from build123d import *

# Parameters (mm, degrees)
ESTRUSIONE_ESTRUSIONE1_DEPTH = 1
ESTRUSIONE_ESTRUSIONE2_DEPTH = 1.5
SCHIZZO4_W                   = 20.34
SCHIZZO4_H                   = 2.54
TAGLIO_ESTRUSIONE1_DEPTH     = 1.5
SCHIZZO5_R                   = 1.25
TAGLIO_ESTRUSIONE2_DEPTH     = 10


with BuildPart() as part:
    # Schizzo2 → Estrusione-Estrusione1 (new body)
    with BuildSketch(Plane(origin=(0, 0, 0), x_dir=(1, 0, 0), z_dir=(0, 1, 0))):
        with BuildLine():
            Line((-3, 0), (-31, 0))
            ThreePointArc((-31, 0), (-33.121320344, 0.878679656), (-34, 3))
            Line((-34, 3), (-34, 47))
            ThreePointArc((-34, 47), (-33.121320344, 49.121320344), (-31, 50))
            Line((-31, 50), (-3, 50))
            ThreePointArc((-3, 50), (-0.878679656, 49.121320344), (0, 47))
            Line((0, 47), (0, 3))
            ThreePointArc((0, 3), (-0.878679656, 0.878679656), (-3, 0))
        make_face()
        with BuildLine():
            Line((-27, 43.75), (-7, 43.75))
            ThreePointArc((-7, 43.75), (-3.464466094, 42.285533906), (-2, 38.75))
            Line((-2, 38.75), (-2, 11.45))
            ThreePointArc((-2, 11.45), (-3.464466094, 7.914466094), (-7, 6.45))
            Line((-7, 6.45), (-27, 6.45))
            ThreePointArc((-27, 6.45), (-30.535533906, 7.914466094), (-32, 11.45))
            Line((-32, 11.45), (-32, 38.75))
            ThreePointArc((-32, 38.75), (-30.535533906, 42.285533906), (-27, 43.75))
        make_face(mode=Mode.SUBTRACT)
    extrude(amount=ESTRUSIONE_ESTRUSIONE1_DEPTH)

    # Schizzo3 → Estrusione-Estrusione2 (add)
    with BuildSketch(Plane(origin=(0, 1, 0), x_dir=(1, 0, 0), z_dir=(0, 1, 0))):
        with BuildLine():
            Line((-30, 52), (-4, 52))
            ThreePointArc((-4, 52), (0.242640687, 50.242640687), (2, 46))
            Line((2, 46), (2, 4))
            ThreePointArc((2, 4), (0.242640687, -0.242640687), (-4, -2))
            Line((-4, -2), (-30, -2))
            ThreePointArc((-30, -2), (-34.242640687, -0.242640687), (-36, 4))
            Line((-36, 4), (-36, 46))
            ThreePointArc((-36, 46), (-34.242640687, 50.242640687), (-30, 52))
        make_face()
        with BuildLine():
            Line((-27, 6.45), (-7, 6.45))
            ThreePointArc((-7, 6.45), (-3.464466094, 7.914466094), (-2, 11.45))
            Line((-2, 11.45), (-2, 38.75))
            ThreePointArc((-2, 38.75), (-3.464466094, 42.285533906), (-7, 43.75))
            Line((-7, 43.75), (-27, 43.75))
            ThreePointArc((-27, 43.75), (-30.535533906, 42.285533906), (-32, 38.75))
            Line((-32, 38.75), (-32, 11.45))
            ThreePointArc((-32, 11.45), (-30.535533906, 7.914466094), (-27, 6.45))
        make_face(mode=Mode.SUBTRACT)
    extrude(amount=ESTRUSIONE_ESTRUSIONE2_DEPTH)

    # Schizzo4 → Taglio-Estrusione1 (cut)
    with BuildSketch(Plane.XZ):
        with Locations((-16.995, -47.1)):
            Rectangle(SCHIZZO4_W, SCHIZZO4_H)
    extrude(amount=-TAGLIO_ESTRUSIONE1_DEPTH, mode=Mode.SUBTRACT)

    # Schizzo5 → Taglio-Estrusione2 (cut)
    with BuildSketch(Plane(origin=(0, 2.5, 0), x_dir=(1, 0, 0), z_dir=(0, 1, 0))):
        with Locations(Location((-30, 46.5, 0), (0, 0, 270))):
            Circle(SCHIZZO5_R)
        with Locations(Location((-4, 46.5, 0), (0, 0, 270))):
            Circle(SCHIZZO5_R)
        with Locations(Location((-4, 3.5, 0), (0, 0, 270))):
            Circle(SCHIZZO5_R)
        with Locations(Location((-30, 3.5, 0), (0, 0, 270))):
            Circle(SCHIZZO5_R)
    extrude(amount=-TAGLIO_ESTRUSIONE2_DEPTH, mode=Mode.SUBTRACT)


solid = part.part
The listing builds one solid part. Answer for the finished solid, in the listing's coordinates (mm). A direction names the side the tool comes from. Round coordinates to 2 decimals unless told otherwise and drop trailing zeros. Write each loop counter-clockwise with the first axis right and the second up, starting at its lowest first coordinate (ties: lowest second). Pieces come first, ordered by that corner, then holes. Notation, with made-up numbers: M 46,68 L 83,68 A25 cw 83,84 Z; hole C 12.25,-24 d10. An arc over 180 degrees is marked long. Write each question's results on one line, items separated by ' | '. Start each with the question number.
Item 1: Flat-ended cylindrical pins translate along their axes: pin 1 Ø1.5 at (x, z) = (-4, -3.5) entering from -Y; pin 2 Ø0.8 at (y, z) = (0.5, -27) entering from +X. Find the tip coordinate at first contact, or state that the pin passes through.
Item 2: A cutting plane is placed at B-B on x = -12. Write down the section's boundary in (y, z).
Item 3: A cutting plane is placed at A-A on z = -31. Write down the section's boundary in (x, y).
Item 4: For a pull along X with two mould halves and no side action, classify faces 5 (the face through (-5.109, 1.268, -2.923)), 6 (the face through (-33.14, 0.49, -49.1)), 7 (the face through (1, 1, -25)) as pulls with the +X half, pulls with the -X half, needs draft (parallel to the pull), parting line crosses it, or undercut.
Item 5: A cutting plane is placed at C-C on z = -10.5. Write down the section's boundary in (x, y), and give its area (3 significant figures).
Item 6: Straight lines are drawn through the part: L1, parallel to Z at x = -15, y = 0.5; L2, parallel to X at y = 0.9, z = -46.5 (3 decimals); L3, parallel to X at y = 1.3, z = -3.5. For each, find the intervals that lie inside material, in ascending order. Write a range as [from, to].
Item 7: For faces 1 (the face through (-30.57, 1.23, -7.95)), 2 (the face through (-17, 1.5, -47)), 3 (the face through (-0.9, 0.49, -49.14)), 4 (the face through (-33.1, 0.49, -0.86)), determine the directions among +Z, -Z, +X, -X, +Y, -Y from which every point of the face is accessible in a straight line to the end or side of a thin tool.
Check sheet entries:
1) pin 1: through | pin 2: x = 0
2) outline: M 0,-50 L 1,-50 L 1,-52 L 2.5,-52 L 2.5,-43.75 L 0,-43.75 L 0,-45.83 L 1.5,-45.83 L 1.5,-48.37 L 0,-48.37 Z; M 0,-6.45 L 2.5,-6.45 L 2.5,2 L 1,2 L 1,0 L 0,0 Z
3) outline: M -36,1 L -34,1 L -34,0 L -32,0 L -32,2.5 L -36,2.5 Z; M -2,0 L 0,0 L 0,1 L 2,1 L 2,2.5 L -2,2.5 Z
4) face 5: undercut | face 6: pulls with the -X half | face 7: needs draft
5) outline: M -36,1 L -34,1 L -34,0 L -31.91,0 L -31.91,2.5 L -36,2.5 Z; M -2.09,0 L 0,0 L 0,1 L 2,1 L 2,2.5 L -2.09,2.5 Z | area: 16.5 mm²
6) L1: [-50, -48.37], [-45.83, -43.75], [-6.45, 0] | L2: [-34, -31.25], [-28.75, -27.165], [-6.825, -5.25], [-2.75, 0] | L3: [-35.98, -31.25], [-28.75, -5.25], [-2.75, 1.98]
7) face 1: +Y, -Y | face 2: -Y | face 3: -Z, +X, -Y | face 4: +Z, -X, -Y
